from build123d import *

# Parameters (mm, degrees)
SKETCH1_W           = 38.1
SKETCH1_H           = 35.56
BOSS_EXTRUDE2_DEPTH = 19.05
SKETCH2_R           = 7.9375
CUT_EXTRUDE1_DEPTH  = 5.08
SKETCH3_R           = 4.7625
CUT_EXTRUDE2_DEPTH  = 43.063657711
SKETCH4_R           = 1.5875
CUT_EXTRUDE3_DEPTH  = 45.612986898
SKETCH5_W           = 11.1125
SKETCH5_H           = 10.16
CUT_EXTRUDE4_DEPTH  = 45.612986898
CUT_EXTRUDE5_DEPTH  = 5.08


with BuildPart() as part:
    # Sketch1 → Boss-Extrude2 (new, symmetric)
    with BuildSketch(Plane.XY):
        Rectangle(SKETCH1_W, SKETCH1_H)
    extrude(amount=BOSS_EXTRUDE2_DEPTH, both=True)

    # Sketch2 → Cut-Extrude1 (cut)
    with BuildSketch(Plane.XY.offset(19.05)):
        Circle(SKETCH2_R)
    cut_extrude1 = extrude(amount=-CUT_EXTRUDE1_DEPTH, mode=Mode.SUBTRACT)

    # Sketch3 → Cut-Extrude2 (cut, through all)
    with BuildSketch(Plane.XY.offset(13.97)):
        Circle(SKETCH3_R)
    extrude(amount=-CUT_EXTRUDE2_DEPTH, mode=Mode.SUBTRACT)

    # Mirror1: Cut-Extrude1 across plane
    add(cut_extrude1.mirror(Plane.XY), mode=Mode.SUBTRACT)

    # Sketch4 → Cut-Extrude3 (cut, through all)
    with BuildSketch(Plane.XZ.offset(17.78)):
        with Locations(Location((13.97, 11.43, 0), (0, 0, 270))):
            Circle(SKETCH4_R)
        with Locations(Location((13.97, -11.43, 0), (0, 0, 270))):
            Circle(SKETCH4_R)
        with Locations(Location((-13.97, -11.43, 0), (0, 0, 270))):
            Circle(SKETCH4_R)
        with Locations(Location((-13.97, 11.43, 0), (0, 0, 270))):
            Circle(SKETCH4_R)
    extrude(amount=-CUT_EXTRUDE3_DEPTH, mode=Mode.SUBTRACT)

    # Sketch5 → Cut-Extrude4 (cut, through all)
    with BuildSketch(Plane(origin=(0, 17.78, 0), x_dir=(1, 0, 0), z_dir=(0, 1, 0))):
        with Locations((13.49375, 0)):
            Rectangle(SKETCH5_W, SKETCH5_H)
    cut_extrude4 = extrude(amount=-CUT_EXTRUDE4_DEPTH, mode=Mode.SUBTRACT)

    # Mirror2: Cut-Extrude4 across plane
    add(cut_extrude4.mirror(Plane(origin=(0, 0, 0), x_dir=(0, 0, 1), z_dir=(1, 0, 0))), mode=Mode.SUBTRACT)

    # Sketch6 → Cut-Extrude5 (cut)
    with BuildSketch(Plane(origin=(0, 17.78, 0), x_dir=(1, 0, 0), z_dir=(0, 1, 0))):
        Polygon((-19.05, 5.08), (-7.9375, 5.08), (-7.9375, -5.08), (-19.05, -5.08), (-19.05, -19.05), (19.05, -19.05), (19.05, -5.08), (7.9375, -5.08), (7.9375, 5.08), (19.05, 5.08), (19.05, 19.05), (-19.05, 19.05), align=None)
    extrude(amount=-CUT_EXTRUDE5_DEPTH, mode=Mode.SUBTRACT)


solid = part.part
Work out the finished part from the listing and answer in its coordinate system (mm). A direction names the side the tool comes from. Round coordinates to 2 decimals unless told otherwise and drop trailing zeros. Write each loop counter-clockwise with the first axis right and the second up, starting at its lowest first coordinate (ties: lowest second). Pieces come first, ordered by that corner, then holes. Notation, with made-up numbers: (10, 75) -> (45, 75) arc R36 cw to (45, 114) -> close; hole circle Ø11 at (-29, -20.75). An arc over 180 degrees is marked (long way). Answer as CSV lines item,"result". Start each with the question number.
(1) The mould has two halves that part along X. Classify faces 4 (the flat face through (-19.05, -3, 12)), 5 (the flat face through (0, -5, -13.97)), 6 (the flat face through (-13, -2, -5.08)): +X half, -X half, draft (parallel to the pull), parting line (faces both ways), or undercut.
(2) Each of these flat-tipped pins is pushed along its axis until it touches: pin 1 (6 mm diameter, centred on x = -2, y = -3.5, fed in from +Z); pin 2 (5 mm diameter, centred on x = -1.5, y = 3.5, fed in from -Z). Where does it stop, or does it pass through?
(3) The part is cut by section D-D, the plane x = 13.97. Give the vertices of the cut face in (y, z), then the cut area to 3 significant figures.
(4) Find the intervals of material crossed by probe 1 along Z at (x, y) = (13, -9); probe 2 along Z at (x, y) = (-16, 4.5); probe 3 along X at (y, z) = (-0.5, 11), in increasing order.
(5) The part is cut by section B-B, the plane z = -11.43. Give the number of separate pieces and of enclosed holes in the cut face, then the cut area to 3 significant figures.
(6) A tool of negligible diameter and unlimited length cuts with its end or side. For faces 1 (the cylindrical face through (-1.72, -7.75, 16.55)), 2 (the cylindrical face through (-1.72, -7.75, -16.55)), 3 (the flat face through (-7.938, -2, 0)), from which of +Z, -Z, +X, -X, +Y, -Y can it reach the whole face along a straight path? Write none if from no direction.
(7) The part is cut by section A-A, the plane x = -11. Give the vertices of the cut face in (y, z).
Output values:
1,face 4,"-X half"
1,face 5,"undercut"
1,face 6,"draft"
2,pin 1,"stops at z = 13.97"
2,pin 2,"stops at z = -13.97"
3,outline,"(-17.78, -19.05) -> (12.7, -19.05) -> (12.7, -13.02) -> (-17.78, -13.02) -> close; (-17.78, -9.84) -> (12.7, -9.84) -> (12.7, -5.08) -> (-17.78, -5.08) -> close; (-17.78, 5.08) -> (12.7, 5.08) -> (12.7, 9.84) -> (-17.78, 9.84) -> close; (-17.78, 13.02) -> (12.7, 13.02) -> (12.7, 19.05) -> (-17.78, 19.05) -> close"
3,area,"658 mm²"
4,probe 1,"z = -19.05 to -12.69, -10.17 to -5.08, 5.08 to 10.17, 12.69 to 19.05"
4,probe 2,"z = -19.05 to -5.08, 5.08 to 19.05"
4,probe 3,"x = -19.05 to -15.5, -12.44 to -4.74, 4.74 to 12.44, 15.5 to 19.05"
5,separate pieces,"3"
5,enclosed holes,"1"
5,area,"896 mm²"
6,face 1,"+Z"
6,face 2,"-Z"
6,face 3,"-X, +Y, -Y"
7,outline,"(-17.78, -19.05) -> (12.7, -19.05) -> (12.7, -5.08) -> (-17.78, -5.08) -> close; (-17.78, 5.08) -> (12.7, 5.08) -> (12.7, 19.05) -> (-17.78, 19.05) -> close"
